The listing builds one solid part. Answer for the finished solid, in the listing's coordinates (mm). A direction names the side the tool comes from. Coordinates: 2 decimals unless noted, no trailing zeros. Order: outer loops, then holes, each group sorted by start corner. A loop starts at its lowest first (then second) coordinate and runs counter-clockwise, first axis right, second up. Notation, with made-up numbers: (85, -16) -> (106, -16) arc R22 ccw to (106, 19) -> close; hole circle Ø3 at (-33, 43). An arc over 180 degrees is marked (long way). Return JSON: item names as keys, results as strings.
```python
from build123d import *

# Parameters (mm, degrees)
F0_W     = 110
F0_H     = 110
F1_DEPTH = 30
F2_W     = 100
F2_H     = 100
F3_DEPTH = 23
F4_W     = 18
F4_H     = 7
F5_DEPTH = 10
F6_W     = 18
F6_H     = 7
F7_DEPTH = 10
F8_R     = 1.85
F9_DEPTH = 7


with BuildPart() as f1:
    # F0 (on Front) → F1 (new body)
    with BuildSketch(Plane.XZ):
        Rectangle(F0_W, F0_H)
    extrude(amount=F1_DEPTH)

    # F2 (on face) → F3 (cut)
    with BuildSketch(Plane.XZ.offset(30)):
        Rectangle(F2_W, F2_H)
    extrude(amount=-F3_DEPTH, mode=Mode.SUBTRACT)

    # F4 (on face) → F5 (cut)
    with BuildSketch(Plane.YZ.offset(55)):
        with Locations((-16, 39.5)):
            Rectangle(F4_W, F4_H)
    extrude(amount=-F5_DEPTH, mode=Mode.SUBTRACT)

    # F6 (on face) → F7 (cut)
    with BuildSketch(Plane(origin=(-55, 0, 0), x_dir=(0, -1, 0), z_dir=(-1, 0, 0))):
        with Locations((16, 40.5)):
            Rectangle(F6_W, F6_H)
    extrude(amount=-F7_DEPTH, mode=Mode.SUBTRACT)

    # F8 (on face) → F9 (cut)
    with BuildSketch(Plane.XZ.offset(30)):
        with Locations((-36.546465, 52.5)):
            Circle(F8_R)
        with Locations((36.546465, 52.5)):
            Circle(F8_R)
        with Locations((-36.546465, -52.5)):
            Circle(F8_R)
        with Locations((36.546465, -52.5)):
            Circle(F8_R)
    extrude(amount=-F9_DEPTH, mode=Mode.SUBTRACT)


solid = f1.part
```
Item 1: Find the intervals of material crossed by probe 1 along Z at (x, y) = (-41, -19.5); probe 2 along Y at (x, z) = (-18, 36.5), in increasing order.
Answer list:
{"probe 1": "-55 to -50, 50 to 55", "probe 2": "-7 to 0"}
Item 2: Which of the six approach directions +Z, -Z, +X, -X, +Y, -Y give full straight-line access (tool end or side, diameter ignored) to faces 4 (the flat face through (-53, -16, 44)), 5 (the flat face through (53, -16, 36)), 6 (the flat face through (-1, -19, -50)), 7 (the flat face through (0, -30, 53)), 8 (the flat face through (55, -15, -1))?
Answer list:
{"face 4": "-X", "face 5": "+X", "face 6": "-Y", "face 7": "+Z, -Z, +X, -X, -Y", "face 8": "+Z, -Z, +X, +Y, -Y"}
Item 3: The part is cut by section C-C on z = 41.5. Determine the outline of the cut face in (x, y).
Answer list:
{"outline": "(-55, -30) -> (-50, -30) -> (-50, -25) -> (-55, -25) -> close; (-55, -7) -> (55, -7) -> (55, 0) -> (-55, 0) -> close; (50, -30) -> (55, -30) -> (55, -25) -> (50, -25) -> close"}
Item 4: Determine the mould class of faces 1 (the flat face through (37, -23, 53)), 2 (the cylindrical face through (-36.948, -26.549, 50.694)), 3 (the flat face through (-53, -16, 37)) for opening direction Y: pulls with the +Y half, pulls with the -Y half, needs draft (parallel to the pull), parting line crosses it, or undercut.
Answer list:
{"face 1": "pulls with the -Y half", "face 2": "needs draft", "face 3": "undercut"}
Item 5: The part is cut by section D-D on x = 19.5. Determine the outline of the cut face in (y, z).
Answer list:
{"outline": "(-30, -55) -> (0, -55) -> (0, 55) -> (-30, 55) -> (-30, 50) -> (-7, 50) -> (-7, -50) -> (-30, -50) -> close"}
Item 6: The part is cut by section A-A on z = 52.5. Determine the outline of the cut face in (x, y).
Answer list:
{"outline": "(-55, -30) -> (-38.4, -30) -> (-38.4, -23) -> (-34.7, -23) -> (-34.7, -30) -> (34.7, -30) -> (34.7, -23) -> (38.4, -23) -> (38.4, -30) -> (55, -30) -> (55, 0) -> (-55, 0) -> close"}
Item 7: The part is cut by section B-B on y = -18. Determine the outline of the cut face in (x, z), plus the area to 3 significant figures.
Answer list:
{"outline": "(-55, -55) -> (55, -55) -> (55, 36) -> (50, 36) -> (50, -50) -> (-50, -50) -> (-50, 37) -> (-55, 37) -> close; (-55, 44) -> (-50, 44) -> (-50, 50) -> (50, 50) -> (50, 43) -> (55, 43) -> (55, 55) -> (-55, 55) -> close", "area": "2,030 mm2"}
Item 8: Flat-ended cylindrical pins translate along their axes: pin 1 (1 mm diameter, centred on x = -32.5, z = 30.5, fed in from -Y); pin 2 (1.9 mm diameter, centred on x = -36, z = -53, fed in from -Y). Find the tip coordinate at first contact, or state that the pin passes through.
Answer list:
{"pin 1": "y = -7", "pin 2": "y = -23"}
